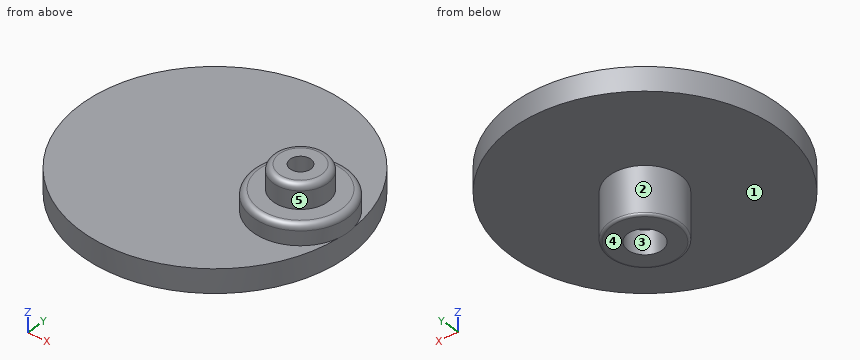
```python
from build123d import *

# Parameters (mm, degrees)
ESQUISSE1_R                  = 11.25
BOSS_EXTRU_1_DEPTH           = 2
ESQUISSE2_R                  = 4
BOSS_EXTRU_2_DEPTH           = 1.7
ESQUISSE3_R                  = 2.3
BOSS_EXTRU_3_DEPTH           = 2
CONG_1_R                     = 0.5
ESQUISSE4_R                  = 3
BOSS_EXTRU_4_DEPTH           = 4
ESQUISSE5_R                  = 1.45
ENL_V_MAT_EXTRU_1_DEPTH      = 2
TROU_TARAUD_M2_2X0_451_D     = 1.75
TROU_TARAUD_M2_2X0_451_DEPTH = 5
TROU_TARAUD_M2_2X0_451_TIP   = 0.525753042
CONG_2_R                     = 0.2


with BuildPart() as part:
    # Esquisse1 → Boss.-Extru.1 (new body)
    with BuildSketch(Plane.XY):
        Circle(ESQUISSE1_R)
    extrude(amount=BOSS_EXTRU_1_DEPTH)

    # Esquisse2 → Boss.-Extru.2 (add)
    with BuildSketch(Plane.XY.offset(2)):
        with Locations(Location((7.3, 0, 0), (0, 0, 348.723074946))):
            Circle(ESQUISSE2_R)
    extrude(amount=BOSS_EXTRU_2_DEPTH)

    # Esquisse3 → Boss.-Extru.3 (add)
    with BuildSketch(Plane.XY.offset(3.7)):
        with Locations((7.3, 0)):
            Circle(ESQUISSE3_R)
    extrude(amount=BOSS_EXTRU_3_DEPTH)

    # Congé1
    cong_1_edges = [part.edges().sort_by_distance(p)[0] for p in [
        (5, 0, 5.7),
        (3.377226027, 0.782204807, 3.7),
    ]]
    fillet(cong_1_edges, radius=CONG_1_R)

    # Esquisse4 → Boss.-Extru.4 (add)
    with BuildSketch(Plane(origin=(0, 0, 0), x_dir=(-1, 0, 0), z_dir=(0, 0, -1))):
        Circle(ESQUISSE4_R)
    extrude(amount=BOSS_EXTRU_4_DEPTH)

    # Esquisse5 → Enlèv. mat.-Extru.1 (cut)
    with BuildSketch(Plane(origin=(0, 0, -4), x_dir=(-1, 0, 0), z_dir=(0, 0, -1))):
        Circle(ESQUISSE5_R)
    extrude(amount=-ENL_V_MAT_EXTRU_1_DEPTH, mode=Mode.SUBTRACT)

    # Trou taraudé M2.2x0.451
    with Locations(Plane.XY.offset(5.7)):
        with Locations((7.3, 0)):
            Hole(TROU_TARAUD_M2_2X0_451_D / 2, depth=TROU_TARAUD_M2_2X0_451_DEPTH)
            with Locations((0, 0, -(TROU_TARAUD_M2_2X0_451_DEPTH + TROU_TARAUD_M2_2X0_451_TIP / 2))):  # 118° drill point
                Cone(0, TROU_TARAUD_M2_2X0_451_D / 2, TROU_TARAUD_M2_2X0_451_TIP, mode=Mode.SUBTRACT)

    # Congé2
    cong_2_edges = [part.edges().sort_by_distance(p)[0] for p in [
        (3, 0, -4),
    ]]
    fillet(cong_2_edges, radius=CONG_2_R)


solid = part.part
```
Design review of the part built by this model. Coordinates are the model's own, in mm. Face numbers are marked on the shaded views. A direction names the side the tool comes from. Give positions to 0.01 mm unless a question says otherwise; leave off trailing zeros. Loops run counter-clockwise (first coordinate to the right, second up) from the corner with the lowest first, then second, coordinate; pieces in that order, holes last. Notation, with made-up numbers: (4, 25.5) -> (57, 25.5) arc R7 ccw to (57, 32.5) -> close; hole circle Ø5 at (-31.5, 7). An arc over 180 degrees is marked (long way). Write each question's results on one line, items separated by ' | '.
Q1. Take a section at B-B, the plane z = 1.5. Write out the cut boundary in (x, y) (3 decimals), plus the area to 3 significant figures.
Reply:
outline: circle Ø22.5 at (0, 0); hole circle Ø1.75 at (7.3, 0) | area: 395 mm²
Q2. For pin 1 Ø1 at (x, z) = (2.5, -2) entering from -Y; pin 2 Ø11 at (x, y) = (-4, 5) entering from +Z; pin 3 Ø3 at (x, z) = (-7, 0.5) entering from +Y; pin 4 Ø4 at (y, z) = (6, 4.5) entering from -X, all flat-tipped, find the tip position at first contact; note any pin that passes through.
Reply:
pin 1: stops at y = -2.24 | pin 2: stops at z = 2 | pin 3: stops at y = 9.81 | pin 4: passes through
Q3. The part is to be moulded in two halves that separate along Y. For the marked faces 1, 2 and 3, say which applies: +Y half, -Y half, draft (parallel to the pull), parting line (faces both ways), or undercut.
Reply:
face 1: draft | face 2: parting line | face 3: undercut
Q4. Machinability: for the marked faces 4 and 5, which of the approach directions +Z, -Z, +X, -X, +Y, -Y give a long, thin tool a straight path to every point of the face, cutting with its end or side? Answer none if there is none.
Reply:
face 4: -Z, +X, -X, +Y, -Y | face 5: +Z
Q5. Wall thickness on L1, parallel to X at y = 0, z = 2.75 (3 decimals); L2, parallel to Y at x = 7.3, z = 4.35 (3 decimals); L3, parallel to Y at x = 7.3, z = 2.55 (3 decimals): over which ranges is each line inside the solid? List them lowest first.
Reply:
L1: x = 3.3 to 6.425, 8.175 to 11.3 | L2: y = -2.3 to -0.875, 0.875 to 2.3 | L3: y = -4 to -0.875, 0.875 to 4
Q6. Take a section at D-D, the plane z = -1. Write out the cut boundary in (x, y), plus the area to 3 significant figures.
Reply:
outline: circle Ø6 at (0, 0) | area: 28.3 mm²
Q7. Take a section at A-A, the plane x = 0. Write out the cut boundary in (y, z).
Reply:
outline: (-11.25, 0) -> (-3, 0) -> (-3, -3.8) arc R0.2 ccw to (-2.8, -4) -> (-1.45, -4) -> (-1.45, -2) -> (1.45, -2) -> (1.45, -4) -> (2.8, -4) arc R0.2 ccw to (3, -3.8) -> (3, 0) -> (11.25, 0) -> (11.25, 2) -> (-11.25, 2) -> close
Q8. Take a section at C-C, the plane y = -9. Write out the cut boundary in (x, z).
Reply:
outline: (-6.75, 0) -> (6.75, 0) -> (6.75, 2) -> (-6.75, 2) -> close
